Input: dimensioned drawing with shaded views. Units: mm. Origin: part minimum x, y, z. A direction names the side the tool comes from. Give positions to 0.01 mm unless a question says otherwise; leave off trailing zeros. Loops run counter-clockwise (first coordinate to the right, second up) from the corner with the lowest first, then second, coordinate; pieces in that order, holes last. Notation, with made-up numbers: (66, -22) -> (87, -22) arc R22 ccw to (87, -2) -> close; hole circle Ø10 at (-38, 63.5). An arc over 180 degrees is marked (long way). Answer in a Markdown table with one row per item. Add a question column.
1) Section query C-C (x = 35). Return the cut outline in (y, z), plus the area to 3 significant figures.
2) Line query: line 1 (Z direction, x = 12.5, y = 3.25); line 2 (X direction, y = 4, z = 3.5); line 3 (Z direction, x = 12.5, y = 6.5). Output: solid intervals per line, ascending. Write a range as from..to.
3) Section query A-A (y = 8.75). Return the cut outline in (x, z), plus the area to 3 significant figures.
4) Access query for the marked faces 4 and 5. Directions: +Z, -Z, +X, -X, +Y, -Y. A direction counts if a zero-diameter tool reaches every point of the face in a straight line with its end or side. Return the directions, or none.
5) Section query B-B (z = 4.5). Return the cut outline in (x, y).
6) First-contact query: P1, Ø1, axis at x = 15, z = 10, coming from the +Y side; P2, Ø1.8, axis at x = 12.5, z = 23.5, coming from the -Y side. Flat tips, straight axial feed; report the tip coordinate or a pass-through.
7) Draft query along Y for the marked faces 1, 2 and 3. Return one class per face: +Y half, -Y half, draft (parallel to the pull), parting line (faces both ways), or undercut.
8) Section query D-D (y = 1.25). Return the cut outline in (x, z), plus the area to 3 significant figures.
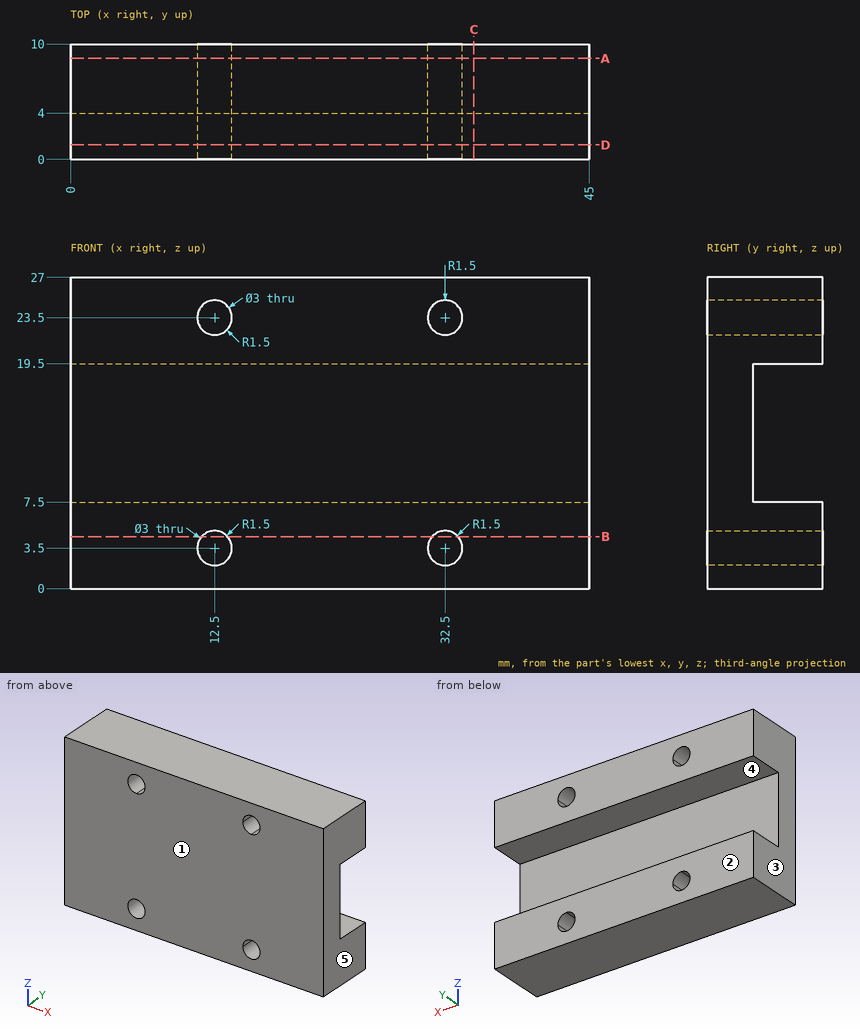
Evaluation:
| question | item | result |
|---|---|---|
| 1 | outline | (0, 0) -> (10, 0) -> (10, 7.5) -> (4, 7.5) -> (4, 19.5) -> (10, 19.5) -> (10, 27) -> (0, 27) -> close |
| 1 | area | 198 mm² |
| 2 | line 1 | 0..2, 5..22, 25..27 |
| 2 | line 2 | 0..11, 14..31, 34..45 |
| 2 | line 3 | 0..2, 5..7.5, 19.5..22, 25..27 |
| 3 | outline | (0, 0) -> (45, 0) -> (45, 7.5) -> (0, 7.5) -> close; (0, 19.5) -> (45, 19.5) -> (45, 27) -> (0, 27) -> close; hole circle Ø3 at (12.5, 3.5); hole circle Ø3 at (12.5, 23.5); hole circle Ø3 at (32.5, 3.5); hole circle Ø3 at (32.5, 23.5) |
| 3 | area | 647 mm² |
| 4 | face 4 | +X, -X, +Y |
| 4 | face 5 | +Z, -Z, +X, +Y, -Y |
| 5 | outline | (0, 0) -> (11.38, 0) -> (11.38, 10) -> (0, 10) -> close; (13.62, 0) -> (31.38, 0) -> (31.38, 10) -> (13.62, 10) -> close; (33.62, 0) -> (45, 0) -> (45, 10) -> (33.62, 10) -> close |
| 6 | P1 | y = 4 |
| 6 | P2 | through |
| 7 | face 1 | -Y half |
| 7 | face 2 | +Y half |
| 7 | face 3 | draft |
| 8 | outline | (0, 0) -> (45, 0) -> (45, 27) -> (0, 27) -> close; hole circle Ø3 at (12.5, 3.5); hole circle Ø3 at (12.5, 23.5); hole circle Ø3 at (32.5, 3.5); hole circle Ø3 at (32.5, 23.5) |
| 8 | area | 1,190 mm² |
